Study the drawing (mm; zero at the part's minimum x, y, z) and answer. Coordinates: 2 decimals unless noted, no trailing zeros. Write each loop counter-clockwise with the first axis right and the second up, starting at its lowest first coordinate (ties: lowest second). Pieces come first, ordered by that corner, then holes. Notation, with made-up numbers: (12.25, 20) - (54.25, 20) arc R23 ccw to (54.25, 32) - close; hole circle Ø9 at (37.25, -4.5). An arc over 180 degrees is marked (long way). One line per item, written item: value.
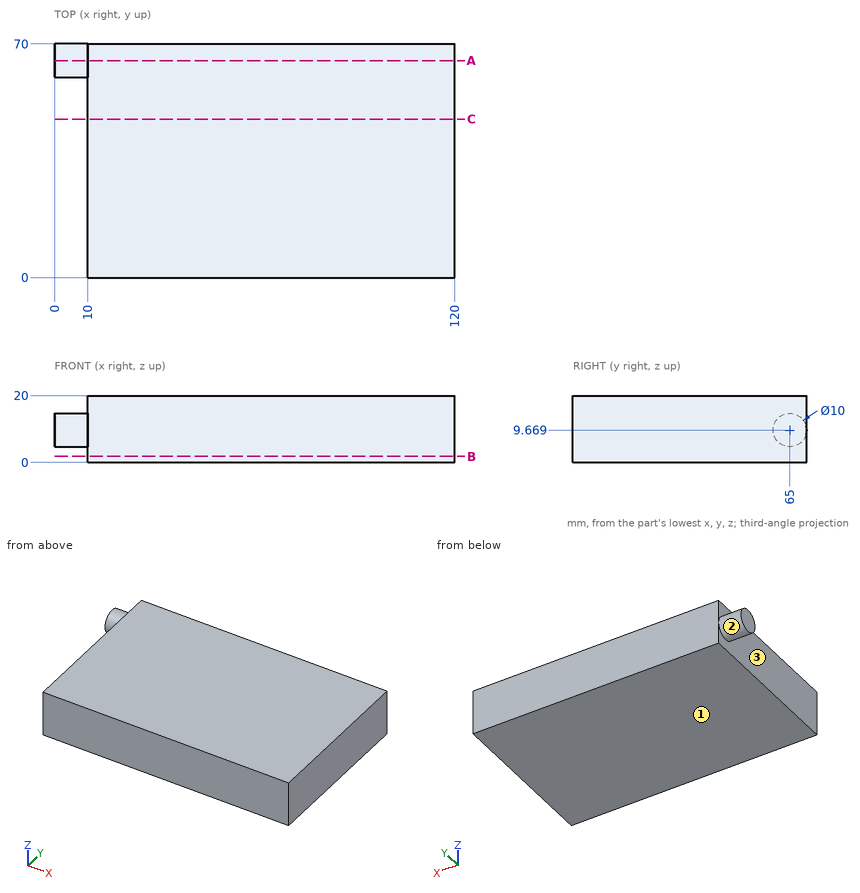
Item 1: Section A-A, the plane y = 65 is taken. Determine the outline of the cut face in (x, z).
Evaluation:
outline: (0, 4.67) - (10, 4.67) - (10, 0) - (120, 0) - (120, 20) - (10, 20) - (10, 14.67) - (0, 14.67) - close
Item 2: Determine the mould class of the marked faces 1, 2 and 3 for opening direction Z: +Z half, -Z half, draft (parallel to the pull), parting line (faces both ways), or undercut.
Evaluation:
face 1: -Z half
face 2: parting line
face 3: draft
Item 3: Section B-B, the plane z = 1.75 is taken. Determine the outline of the cut face in (x, y), then the cut area to 3 significant figures.
Evaluation:
outline: (10, 0) - (120, 0) - (120, 70) - (10, 70) - close
area: 7,700 mm2
Item 4: Consider probe 1 along X at (y, z) = (56.5, 6). Determine where the line is inside the solid, lowest interval first.
Evaluation:
probe 1: x = 10 to 120
Item 5: Given pin 1 (1 mm diameter, centred on x = 57, y = 57.5, fed in from -Z); pin 2 (4 mm diameter, centred on y = 29.5, z = 16, fed in from -X), each flat-ended and moving along its own axis, determine where each tip first touches the part or whether it passes through.
Evaluation:
pin 1: stops at z = 0
pin 2: stops at x = 10
Item 6: Section C-C, the plane y = 47.5 is taken. Determine the outline of the cut face in (x, z).
Evaluation:
outline: (10, 0) - (120, 0) - (120, 20) - (10, 20) - close
